```python
from build123d import *

# Parameters (mm, degrees)
EXTRUDE_1_DEPTH             = 130
HOLE_WIZARD_M3_2_AT_2_COUNT = 2
HOLE_WIZARD_M3_2_AT_2_PITCH = 80


with BuildPart() as part:
    # ｽｹｯﾁ1 → ﾎﾞｽ - 押し出し1 (new body)
    with BuildSketch(Plane.XY):
        with BuildLine():
            Line((0, 35), (0, 28))
            ThreePointArc((0, 28), (0.878679656, 25.878679656), (3, 25))
            Line((3, 25), (28, 25))
            ThreePointArc((28, 25), (29.414213562, 24.414213562), (30, 23))
            Line((30, 23), (30, 0))
            Line((30, 0), (31, 0))
            Line((31, 0), (31, 23))
            ThreePointArc((31, 23), (30.121320344, 25.121320344), (28, 26))
            Line((28, 26), (3, 26))
            ThreePointArc((3, 26), (1.585786438, 26.585786438), (1, 28))
            Line((1, 28), (1, 35))
            Line((1, 35), (0, 35))
        make_face()
    extrude_1 = extrude(amount=EXTRUDE_1_DEPTH)

    # ｽｹｯﾁ5 → M3 すきま穴2 (revolve, cut)
    with BuildSketch(Plane(origin=(1, 30, 25), x_dir=(0, 0, -1), z_dir=(0, 1, 0))):
        Polygon((0, 0), (0, 10.96137699), (1.6, 10), (1.6, 0), align=None)
    hole_wizard_m3_2 = revolve(axis=Axis((7.35, 30, 25), (-1, 0, 0)), mode=Mode.SUBTRACT)

    # M3 すきま穴2 at 2: M3 すきま穴2 ×2
    with Locations(*[(0, 0, i * HOLE_WIZARD_M3_2_AT_2_PITCH) for i in range(1, HOLE_WIZARD_M3_2_AT_2_COUNT)]):
        add(hole_wizard_m3_2, mode=Mode.SUBTRACT)

    # ﾐﾗｰ2: ﾎﾞｽ - 押し出し1, M3 すきま穴2 across plane
    add(extrude_1.mirror(Plane.ZX))
    add(hole_wizard_m3_2.mirror(Plane.ZX), mode=Mode.SUBTRACT)

    # ﾐﾗｰ2 copy 1 sketch → ﾐﾗｰ2 copy 1 (revolve, cut)
    with BuildSketch(Plane(origin=(1, -30, 105), x_dir=(0, 0, -1), z_dir=(0, -1, 0))):
        Polygon((0, 0), (0, -10.96137699), (1.6, -10), (1.6, 0), align=None)
    revolve(axis=Axis((7.35, -30, 105), (1, 0, 0)), mode=Mode.SUBTRACT)


solid = part.part
```
Geometry: final body of the model. Coordinates: model frame, mm. A direction names the side the tool comes from. Round coordinates to 2 decimals unless told otherwise and drop trailing zeros. Write each loop counter-clockwise with the first axis right and the second up, starting at its lowest first coordinate (ties: lowest second). Pieces come first, ordered by that corner, then holes. Notation, with made-up numbers: M 15.5,48 L 27.5,48 A20 cw 27.5,53 Z; hole C -8.5,27 d6. An arc over 180 degrees is marked long. Answer in a Markdown table with one row per item. Add a question column.
(1) Contact query for flat-ended pins moving along their axis: pin 1 (2 mm diameter, centred on y = 26.5, z = 14.5, fed in from -X); pin 2 (7.5 mm diameter, centred on y = -31, z = 73, fed in from +X); pin 3 (12.5 mm diameter, centred on x = 18.5, z = 45, fed in from +Y). Output: stop coordinate, or through.
(2) Ray query, L1, parallel to Y at x = 0.75, z = 105; L2, parallel to Y at x = 26, z = 111.5; L3, parallel to Y at x = 0.35, z = 25. Return the intervals inside material, ascending.
(3) Cut plane B-B, the plane x = 9. Return the cut outline in (y, z), then the cut area to 3 significant figures.
(4) Draft query along Z for faces 4 (the face through (30.4, 12.8, 0)), 5 (the face through (0, 32, 64)), 6 (the face through (0.51, 28.92, 106.18)), 7 (the face through (30.4, 12.8, 130)). Return one class per face: pulls with the +Z half, pulls with the -Z half, needs draft (parallel to the pull), parting line crosses it, or undercut.
(5) Cut plane A-A, the plane z = 25. Return the cut outline in (x, y), then the cut area to 3 significant figures.
(6) Reachability of faces 1 (the face through (1, -31, 64)), 2 (the face through (0.86, -25.9, 64.09)), 3 (the face through (16, 26, 64)) from +Z, -Z, +X, -X, +Y, -Y: full face, straight path, thin tool, end or side. Return the list, or none.
(7) Cut plane D-D, the plane z = 88.5. Return the cut outline in (x, y), then the cut area to 3 significant figures.
(8) Cut plane C-C, the plane y = -30. Return the cut outline in (x, z), then the cut area to 3 significant figures.
Established:
| question | item | result |
|---|---|---|
| 1 | pin 1 | x = 0.04 |
| 1 | pin 2 | x = 1.15 |
| 1 | pin 3 | y = 26 |
| 2 | L1 | -35 to -31.6, -28.4 to -26.02, 26.02 to 28.4, 31.6 to 35 |
| 2 | L2 | -26 to -25, 25 to 26 |
| 2 | L3 | -35 to -31.6, -28.4 to -26.59, 26.59 to 28.4, 31.6 to 35 |
| 3 | outline | M -26,0 L -25,0 L -25,130 L -26,130 Z; M 25,0 L 26,0 L 26,130 L 25,130 Z |
| 3 | area | 260 mm² |
| 4 | face 4 | pulls with the -Z half |
| 4 | face 5 | needs draft |
| 4 | face 6 | undercut |
| 4 | face 7 | pulls with the +Z half |
| 5 | outline | M 0,-35 L 1,-35 L 1,-31.6 L 0,-31.6 Z; M 0,-28.4 L 1,-28.4 L 1,-28 A2 cw 3,-26 L 28,-26 A3 ccw 31,-23 L 31,23 A3 ccw 28,26 L 3,26 A2 cw 1,28 L 1,28.4 L 0,28.4 L 0,28 A3 ccw 3,25 L 28,25 A2 cw 30,23 L 30,-23 A2 cw 28,-25 L 3,-25 A3 ccw 0,-28 Z; M 0,31.6 L 1,31.6 L 1,35 L 0,35 Z |
| 5 | area | 119 mm² |
| 6 | face 1 | +Z, -Z, +X, -Y |
| 6 | face 2 | +Z, -Z, -X |
| 6 | face 3 | +Z, -Z, +X, +Y |
| 7 | outline | M 0,-35 L 1,-35 L 1,-28 A2 cw 3,-26 L 28,-26 A3 ccw 31,-23 L 31,23 A3 ccw 28,26 L 3,26 A2 cw 1,28 L 1,35 L 0,35 L 0,28 A3 ccw 3,25 L 28,25 A2 cw 30,23 L 30,-23 A2 cw 28,-25 L 3,-25 A3 ccw 0,-28 Z |
| 7 | area | 126 mm² |
| 8 | outline | M 0,0 L 1,0 L 1,23.4 L 0,23.4 Z; M 0,26.6 L 1,26.6 L 1,103.4 L 0,103.4 Z; M 0,106.6 L 1,106.6 L 1,130 L 0,130 Z |
| 8 | area | 124 mm² |
